Read the model definition and answer for the solid it produces. Units are mm, in the model's axes. Round coordinates to 2 decimals unless told otherwise and drop trailing zeros. Loops run counter-clockwise (first coordinate to the right, second up) from the corner with the lowest first, then second, coordinate; pieces in that order, holes last. Notation, with made-up numbers: (-2.5, -13.75) - (36.5, -13.75) arc R3 ccw to (36.5, -8.75) - close; hole circle Ø11 at (-33, 57.5). An arc over 180 degrees is marked (long way). Answer as CSV lines item,"result".
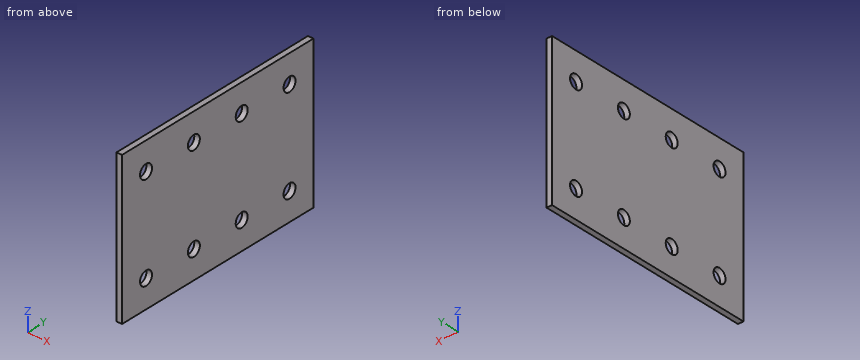
Autodesk Inventor part; units mm, degrees
ref_plane "YZ Plane" through (0, 0, 0) normal (1, 0, 0) x (0, 1, 0)
ref_plane "XZ Plane" through (0, 0, 0) normal (0, 1, 0) x (-1, 0, 0)
ref_plane "XY Plane" through (0, 0, 0) normal (0, 0, 1) x (1, 0, 0)
sketch "Sketch1" plane through (0, 0, 0) normal (1, 0, 0) x (0, 1, 0)
  line L0 (0, 0) -> (-40, 0)
  line L1 (-40, 0) -> (-40, -54.112)
  line L2 (-40, -54.112) -> (0, -54.112)
  line L3 (0, -54.112) -> (0, 0)
  line L4 (-40, -54.112) -> (-40, -44.112)
  line L5 (-40, -44.112) -> (-30, -44.112)
  line L6 (-40, 0) -> (-40, -10)
  line L7 (-40, -10) -> (-30, -10)
  line L8 (0, -10) -> (-10, -10)
  circle A0 centre (-10, -10) radius 2.5
  circle A1 centre (-30, -44.112) radius 2.5
  circle A2 centre (-30, -10) radius 2.5
  line L9 (-40, 0) -> (-60, 0)
  line L10 (-60, 0) -> (-60, -54.112)
  line L11 (-60, -54.112) -> (-40, -54.112)
  line L12 (-40, -54.112) -> (-40, 0)
  line L13 (0, 0) -> (20, 0)
  line L14 (20, 0) -> (20, -54.112)
  line L15 (20, -54.112) -> (0, -54.112)
  line L16 (0, -54.112) -> (0, 0)
  circle A3 centre (10, -10) radius 2.5
  circle A4 centre (-50, -44.112) radius 2.5
  circle A5 centre (-50, -10) radius 2.5
  line L17 (0, -54.112) -> (0, -44.112)
  line L18 (0, -44.112) -> (-10, -44.112)
  circle A6 centre (-10, -44.112) radius 2.5
  circle A7 centre (10, -44.112) radius 2.5
  dimension "d0" = 40
  dimension "d1" = 54.112
  dimension "d2" = 10
  dimension "d3" = 10
  dimension "d4" = 10
  dimension "d5" = 10
  dimension "d6" = 5
  dimension "d8" = 5
  dimension "d9" = 5
  dimension "d10" = 20
  dimension "d11" = 20
  dimension "d14" = 10
  dimension "d15" = 10
  dimension "d16" = 5
extrude "Extrusion1" add sketch "Sketch1" along normal blind 2
properties part number "H-Connector_2020"
1) A cutting plane is placed at B-B, the plane x = 0.7. Count the separate pieces of the cut face and the enclosed holes in it, plus the area to 3 significant figures.
Entries:
separate pieces,"1"
enclosed holes,"8"
area,"4,170 mm^2"
2) Each of these flat-tipped pins is pushed along its axis until it touches: P1, Ø6, axis at y = -30, z = -44.112, coming from the -X side; P2, Ø4.5, axis at y = -10, z = -10, coming from the -X side. Where does it stop, or does it pass through?
Entries:
P1,"stops at x = 0"
P2,"passes through"
3) Find the intervals of material crossed by line 1 (Z direction, x = 1.1, y = -10); line 2 (Y direction, x = 0.2, z = -44); line 3 (Z direction, x = 0.35, y = -9), in increasing order.
Entries:
line 1,"z = -54.11 to -46.61, -41.61 to -12.5, -7.5 to 0"
line 2,"y = -60 to -52.5, -47.5 to -32.5, -27.5 to -12.5, -7.5 to 7.5, 12.5 to 20"
line 3,"z = -54.11 to -46.4, -41.82 to -12.29, -7.71 to 0"
4) A cutting plane is placed at A-A, the plane y = -30. Determine the outline of the cut face in (x, z).
Entries:
outline,"(0, -54.11) - (2, -54.11) - (2, -46.61) - (0, -46.61) - close; (0, -41.61) - (2, -41.61) - (2, -12.5) - (0, -12.5) - close; (0, -7.5) - (2, -7.5) - (2, 0) - (0, 0) - close"
